Geometry: final body of the model. Coordinates: model frame, mm. Give positions to 0.01 mm unless a question says otherwise; leave off trailing zeros. Write each loop counter-clockwise with the first axis right and the second up, starting at its lowest first coordinate (ties: lowest second). Pieces come first, ordered by that corner, then holes. Notation, with made-up numbers: (84.5, 54) -> (104.5, 54) arc R19 ccw to (104.5, 91) -> close; hole circle Ø1 at (5.25, 14). An arc over 180 degrees is marked (long way). Use CSV: the item, a comma, the result in double quotes. Start each with the question number.
1) Section C-C (z = -0.5). Output: boundary loops of the cut face in (x, y), plus the area to 3 significant figures.
2) Draft query along X for faces 1 (the face through (-16.039, 18.566, 0.986)), 2 (the face through (-19, 0, 0)), 3 (the face through (21, 0.3, 0.5)). Return one class per face: pulls with the +X half, pulls with the -X half, needs draft (parallel to the pull), parting line crosses it, or undercut.
3) Section B-B (x = 16.5). Output: boundary loops of the cut face in (y, z), plus the area to 3 significant figures.
4) Section A-A (x = 0). Output: boundary loops of the cut face in (y, z).
5) Contact query for flat-ended pins moving along their axis: P1, Ø2.5, axis at x = 16.5, y = 17.68, coming from the -Z side; P2, Ø2, axis at y = -1.5, z = 1.5, coming from the -X side. Output: stop coordinate, or through.
6) Material intervals for line 1 (Y direction, x = -16.5, z = 1.1); line 2 (Y direction, x = 0, z = -1.7); line 3 (Y direction, x = 16.5, z = 1.45), sorted ascending. Write a range as [from, to].
7) Section D-D (y = -9). Output: boundary loops of the cut face in (x, z), plus the area to 3 significant figures.
Autodesk Inventor part; units mm, degrees
ref_plane "YZ Plane" through (0, 0, 0) normal (1, 0, 0) x (0, 1, 0)
ref_plane "XZ Plane" through (0, 0, 0) normal (0, 1, 0) x (-1, 0, 0)
ref_plane "XY Plane" through (0, 0, 0) normal (0, 0, 1) x (1, 0, 0)
sketch "Sketch1" plane through (0, 0, 0) normal (0, 0, 1) x (1, 0, 0)
  circle A0 centre (0, 0) radius 18.5
  line L0 (-21, 22.5) -> (21, 22.5)
  line L1 (21, 22.5) -> (21, -22.5)
  line L2 (21, -22.5) -> (-21, -22.5)
  line L3 (-21, -22.5) -> (-21, 22.5)
  line L4 (-38, 0) -> (59, 0) construction
  line L5 (0, 34) -> (0, -33) construction
  line L6 (-21, -22.5) -> (21, 22.5) construction
  line L7 (21, -22.5) -> (-21, 22.5) construction
  circle A1 centre (16.5, 17.6786) radius 1
  circle A2 centre (-16.5, 17.6786) radius 1
  circle A3 centre (16.5, -17.6786) radius 1
  circle A4 centre (-16.5, -17.6786) radius 1
  circle A5 centre (0, 0) radius 2
  dimension "d1" = 37
  dimension "d2" = 42
  dimension "d3" = 45
  dimension "d4" = 21
  dimension "d5" = 22.5
  dimension "d6" = 2
  dimension "d7" = 4.5
  dimension "d8" = 4
extrude "Extrusion1" add sketch "Sketch1" along normal blind 3 contours L0 L1 L2 L3
extrude "Extrusion2" add sketch "Sketch1" along normal blind 3 and the other way blind 2 contours A0
fillet "Fillet1" radius 1 4 edges at (15.5, 17.6786, 3) (-17.5, 17.6786, 3) (-17.5, -17.6786, 3) (15.5, -17.6786, 3)
fillet "Fillet2" radius 2 4 edges at (0, 22.5, 3) (21, 0, 3) (0, -22.5, 3) (-21, 0, 3)
fillet "Fillet3" radius 1 8 edges at (-20.4142, 21.9142, 2.4142) (-21, 22.5, 0.5) (20.4142, 21.9142, 2.4142) (21, 22.5, 0.5) (21, -22.5, 0.5) (20.4142, -21.9142, 2.4142) (-20.4142, -21.9142, 2.4142) (-21, -22.5, 0.5)
equation "\"d4\" = 0.5 * d2"
equation "\"d5\" = 0.5 * d3"
properties part number "engine_lid"
Answers follow:
1,outline,"circle Ø37 at (0, 0); hole circle Ø4 at (0, 0)"
1,area,"1,060 mm^2"
2,face 1,"undercut"
2,face 2,"needs draft"
2,face 3,"pulls with the +X half"
3,outline,"(-22.5, 0) -> (-18.68, 0) -> (-18.68, 2) arc R1 ccw to (-19.68, 3) -> (-20.5, 3) arc R2 ccw to (-22.5, 1) -> close; (-16.68, 0) -> (-8.37, 0) -> (-8.37, -2) -> (8.37, -2) -> (8.37, 0) -> (16.68, 0) -> (16.68, 2) arc R1 ccw to (15.68, 3) -> (-15.68, 3) arc R1 ccw to (-16.68, 2) -> close; (18.68, 0) -> (22.5, 0) -> (22.5, 1) arc R2 ccw to (20.5, 3) -> (19.68, 3) arc R1 ccw to (18.68, 2) -> close"
3,area,"154 mm^2"
4,outline,"(-22.5, 0) -> (-18.5, 0) -> (-18.5, -2) -> (-2, -2) -> (-2, 3) -> (-20.5, 3) arc R2 ccw to (-22.5, 1) -> close; (2, -2) -> (18.5, -2) -> (18.5, 0) -> (22.5, 0) -> (22.5, 1) arc R2 ccw to (20.5, 3) -> (2, 3) -> close"
5,P1,"stops at z = 0"
5,P2,"stops at x = -21"
6,line 1,"y = [-22.5, -18.68], [-16.68, 16.68], [18.68, 22.5]"
6,line 2,"y = [-18.5, -2], [2, 18.5]"
6,line 3,"y = [-22.45, -18.68], [-16.68, 16.68], [18.68, 22.45]"
7,outline,"(-21, 0) -> (-16.16, 0) -> (-16.16, -2) -> (16.16, -2) -> (16.16, 0) -> (21, 0) -> (21, 1) arc R2 ccw to (19, 3) -> (-19, 3) arc R2 ccw to (-21, 1) -> close"
7,area,"189 mm^2"
